from build123d import *

# Parameters (mm, degrees)
F1_DEPTH = 25
F4_DEPTH = 1.5


with BuildPart() as f1:
    # F0 (on Front) → F1 (new body)
    with BuildSketch(Plane.XZ):
        with BuildLine():
            ThreePointArc((-33.633865, 7.958327), (-33.19345, 1.238902), (-27.28971, -2.000001))
            Line((-27.28971, -2.000001), (37.262999, -2.000001))
            ThreePointArc((37.262999, -2.000001), (41.024096, -0.903741), (43.607153, 2.041671))
            Line((43.607153, 2.041671), (53.399614, 23.041671))
            ThreePointArc((53.399614, 23.041671), (52.9592, 29.761097), (47.05546, 32.999999))
            Line((47.05546, 32.999999), (-17.49725, 32.999999))
            ThreePointArc((-17.49725, 32.999999), (-21.258347, 31.903739), (-23.841404, 28.958327))
            Line((-23.841404, 28.958327), (-33.633865, 7.958327))
        make_face()
        with BuildLine():
            Line((-30.914941, 6.690472), (-21.122481, 27.690472))
            ThreePointArc((-21.122481, 27.690472), (-20.937767, 28.040303), (-20.719401, 28.370177))
            Line((-20.719401, 28.370177), (-15.790062, 0.999999))
            Line((-15.790062, 0.999999), (-27.28971, 0.999999))
            ThreePointArc((-27.28971, 0.999999), (-30.663276, 2.850801), (-30.914941, 6.690472))
        make_face(mode=Mode.SUBTRACT)
        with BuildLine():
            ThreePointArc((-19.646448, 29.373565), (-18.616566, 29.840199), (-17.49725, 29.999999))
            Line((-17.49725, 29.999999), (-0.946572, 29.999999))
            Line((-0.946572, 29.999999), (-14.5364, 0.999999))
            Line((-14.5364, 0.999999), (-19.646448, 29.373565))
        make_face(mode=Mode.SUBTRACT)
        Polygon((-12.550904, 0.999999), (-0.361492, 27.14028), (4.986644, 0.999999), align=None, mode=Mode.SUBTRACT)
        Polygon((6.905234, 0.999999), (18.372576, 26.895071), (24.439983, 0.999999), align=None, mode=Mode.SUBTRACT)
        with BuildLine():
            ThreePointArc((39.412197, 1.626434), (38.382315, 1.1598), (37.262999, 0.999999))
            Line((37.262999, 0.999999), (26.542474, 0.999999))
            Line((26.542474, 0.999999), (36.609397, 25.947182))
            Line((36.609397, 25.947182), (39.412197, 1.626434))
        make_face(mode=Mode.SUBTRACT)
        Polygon((17.645068, 29.999999), (6.292948, 3.992694), (0.972018, 29.999999), align=None, mode=Mode.SUBTRACT)
        Polygon((36.142338, 29.999999), (25.77013, 4.296282), (19.747559, 29.999999), align=None, mode=Mode.SUBTRACT)
        with BuildLine():
            ThreePointArc((47.05546, 29.999999), (50.429025, 28.149198), (50.680691, 24.309526))
            Line((50.680691, 24.309526), (40.88823, 3.309526))
            Line((40.88823, 3.309526), (38.244829, 29.999999))
            Line((38.244829, 29.999999), (47.05546, 29.999999))
        make_face(mode=Mode.SUBTRACT)
    extrude(amount=F1_DEPTH)

    # F3 (on offset) → F4 (join, symmetric)
    with BuildSketch(Plane.XZ.offset(12.5)):
        Polygon((-32.50682, 4.622142), (-29.003944, -0.644573), (40.218219, 0), (49.982231, 17.865283), (52.67575, 25.833612), (50.543383, 29.761663), (46.615332, 31.894032), (-16.457932, 31.894032), (-21.059362, 30.098353), align=None)
    extrude(amount=F4_DEPTH, both=True)


solid = f1.part
Verification items for the finished model (mm, model axes). A direction names the side the tool comes from. Give positions to 0.01 mm unless a question says otherwise; leave off trailing zeros. Write each loop counter-clockwise with the first axis right and the second up, starting at its lowest first coordinate (ties: lowest second). Pieces come first, ordered by that corner, then holes. Notation, with made-up numbers: M 27,-32 L 70,-32 A20 cw 70,-7 Z; hole C 11.5,20 d6. An arc over 180 degrees is marked long. Put each result on its own line as item: value. Start each with the question number.
1. Section check D-D (x = 32.5). Record the cut outline in (y, z), and give its area (3 significant figures).
2. Go/stop test with flat-tipped pins: pin 1 Ø8 at (x, z) = (18, 10.5) entering from -Y; pin 2 Ø2 at (x, y) = (44.5, -20) entering from -Z; pin 3 Ø1 at (y, z) = (-16.5, 27.5) entering from -X. Record where each tip stops, or that it passes through.
3. Section check A-A (y = -13). Record the cut outline in (x, z).
4. Section check C-C (y = -19.75). Give the number of separate pieces and of enclosed holes in the cut face, and give its area (3 significant figures).
5. Section check B-B (x = -7.5). Record the cut outline in (y, z), and give its area (3 significant figures).
6. Set-up check for faces 1 (the face through (9, -14, 20)), 2 (the face through (43, -5, 30)): record each of +Z, -Z, +X, -X, +Y, -Y from which the full face is reachable in a straight line by a thin tool's end or side.
7. Scan lines: line 1 along Z through (x, y) = (-13, -19.25); line 2 along Z through (x, y) = (17, -8.5); line 3 along Z through (x, y) = (-10.5, -20.5). Record each from-to range of solid material in increasing order. Write a range as [from, to].
Answer list:
1. outline: M -25,-2 L 0,-2 L 0,1 L -11,1 L -11,15.76 L 0,15.76 L 0,20.97 L -11,20.97 L -11,30 L 0,30 L 0,33 L -25,33 L -25,30 L -14,30 L -14,20.97 L -25,20.97 L -25,15.76 L -14,15.76 L -14,1 L -25,1 Z
1. area: 352 mm2
2. pin 1: y = -14
2. pin 2: z = 1.82
2. pin 3: x = -24.75
3. outline: M -33.63,7.96 A7 ccw -27.29,-2 L 37.26,-2 A7 ccw 43.61,2.04 L 53.4,23.04 A7 ccw 47.06,33 L -17.5,33 A7 ccw -23.84,28.96 Z
4. separate pieces: 1
4. enclosed holes: 8
4. area: 993 mm2
5. outline: M -25,-2 L 0,-2 L 0,1 L -11,1 L -11,11.83 L 0,11.83 L 0,16.02 L -11,16.02 L -11,30 L 0,30 L 0,33 L -25,33 L -25,30 L -14,30 L -14,16.02 L -25,16.02 L -25,11.83 L -14,11.83 L -14,1 L -25,1 Z
5. area: 329 mm2
6. face 1: -Y
6. face 2: +Y
7. line 1: [-2, 4.28], [30, 33]
7. line 2: [-2, 1], [23.8, 28.52], [30, 33]
7. line 3: [-2, 1], [5.4, 9.61], [30, 33]
